Work out the finished part from the listing and answer in its coordinate system (mm). A direction names the side the tool comes from. Coordinates: 2 decimals unless noted, no trailing zeros. Order: outer loops, then holes, each group sorted by start corner. A loop starts at its lowest first (then second) coordinate and runs counter-clockwise, first axis right, second up. Notation, with made-up numbers: M -7.5,-28 L 40.5,-28 A16 ccw 40.5,-7 Z; hole C -30,-29 d7. An arc over 180 degrees is marked long. Answer in a Markdown table with one row per item. Add a question column.
Item 1: Flat-ended cylindrical pins translate along their axes: pin 1 Ø4 at (x, z) = (-9, 3.5) entering from -Y; pin 2 Ø4 at (x, y) = (13.5, -1.5) entering from +Z; pin 3 Ø3 at (x, y) = (17.145, 0) entering from -Z; pin 4 Ø2 at (y, z) = (0.5, 11.5) entering from +X (3 decimals). Find the tip coordinate at first contact, or state that the pin passes through.
Item 2: Which of the six approach directions +Z, -Z, +X, -X, +Y, -Y give full straight-line access (tool end or side, diameter ignored) to faces 1 (the face through (-5.3, -0.8, 7.3)), 2 (the face through (-12.657, -3.184, 3.393)), 3 (the face through (-4.191, 0, 10))?
Item 3: The part is cut by section A-A (z = 5.08). Write down the section's boundary in (x, y) (1 decimal), then the cut area to 3 significant figures.
Item 4: The part is cut by section B-B (y = 0.5). Write down the section's boundary in (x, z) (3 decimals).
Item 5: The part is cut by section C-C (x = -8.89). Write down the section's boundary in (y, z), then the cut area to 3 significant figures.
Item 6: The mould has two halves that part along X. Classify faces 4 (the face through (15, 0, 0)), 5 (the face through (-17.145, 0, 5)), 6 (the face through (-4.651, 0.053, 6.773)), 7 (the face through (20.954, -0.084, 5.009)): released by +X, released by -X, zero draft, split by the parting line, or undercut.
Item 7: Consider line 1 (Y direction, x = 17, z = 7.75); line 2 (X direction, y = 0.5, z = 11) (3 decimals); line 3 (Z direction, x = 8.5, y = 2.5). Determine where each line is inside the solid, lowest interval first. Write a range as from..to.
Item 8: The part is cut by section D-D (x = 11.5). Write down the section's boundary in (y, z).
from build123d import *

# Parameters (mm, degrees)
BOSS_EXTRUDE1_DEPTH   = 10.16
F_4_CLEARANCE_HOLE1_D = 3.4544
SKETCH4_R             = 1.905
CUT_EXTRUDE1_DEPTH    = 8.62
CUT_EXTRUDE1_TAPER    = -20
SKETCH5_R             = 4.1275
CUT_EXTRUDE2_DEPTH    = 1.27
SKETCH6_W             = 25.4
SKETCH6_H             = 2.54
BOSS_EXTRUDE2_DEPTH   = 7.62
CUT_EXTRUDE3_DEPTH    = 8.62


with BuildPart() as part:
    # Sketch1 → Boss-Extrude1 (new body)
    with BuildSketch(Plane.XY):
        with BuildLine():
            Line((-17.145, -3.81), (17.145, -3.81))
            ThreePointArc((17.145, -3.81), (20.955, 0), (17.145, 3.81))
            Line((17.145, 3.81), (-17.145, 3.81))
            Line((-17.145, 3.81), (-17.145, -3.81))
        make_face()
    extrude(amount=BOSS_EXTRUDE1_DEPTH)

    # #4 Clearance Hole1 (through all)
    with Locations(Plane.XY.offset(10.16)):
        with Locations((17.145, 0)):
            Hole(F_4_CLEARANCE_HOLE1_D / 2)

    # Sketch4 → Cut-Extrude1 (cut, through all)
    with BuildSketch(Plane(origin=(0, -3.81, 0), x_dir=(1, 0, 0), z_dir=(0, 1, 0))):
        with Locations((-8.89, -5.08)):
            Circle(SKETCH4_R)
    extrude(amount=CUT_EXTRUDE1_DEPTH, taper=CUT_EXTRUDE1_TAPER, mode=Mode.SUBTRACT)

    # Sketch5 → Cut-Extrude2 (cut)
    with BuildSketch(Plane.XZ.offset(3.81)):
        with Locations((-8.89, 5.08)):
            Circle(SKETCH5_R)
    extrude(amount=-CUT_EXTRUDE2_DEPTH, mode=Mode.SUBTRACT)

    # Sketch6 → Boss-Extrude2 (add, through all)
    with BuildSketch(Plane.XZ.offset(3.81)):
        with Locations((-4.445, 11.43)):
            Rectangle(SKETCH6_W, SKETCH6_H)
        with Locations((-4.445, -1.27)):
            Rectangle(SKETCH6_W, SKETCH6_H)
    extrude(amount=-BOSS_EXTRUDE2_DEPTH)

    # Sketch8 → Cut-Extrude3 (cut, through all)
    with BuildSketch(Plane(origin=(0, 3.81, 0), x_dir=(1, 0, 0), z_dir=(0, 1, 0))):
        Polygon((-3.429, -12.7), (-3.429, -7.38452905), (-8.71961162, -4.73922324), (-9.06038838, -5.42077676), (-4.191, -7.85547095), (-4.191, -12.7), align=None)
    extrude(amount=-CUT_EXTRUDE3_DEPTH, mode=Mode.SUBTRACT)


solid = part.part
Reply:
| question | item | result |
|---|---|---|
| 1 | pin 1 | stops at y = -2.54 |
| 1 | pin 2 | stops at z = 10.16 |
| 1 | pin 3 | passes through |
| 1 | pin 4 | stops at x = 8.255 |
| 2 | face 1 | +Y, -Y |
| 2 | face 2 | -Y |
| 2 | face 3 | +Z, +Y, -Y |
| 3 | outline | M -17.1,-3.8 L -13,-3.8 L -13,-2.5 L -11.3,-2.5 L -13.6,3.8 L -17.1,3.8 Z; M -6.5,-2.5 L -4.8,-2.5 L -4.8,-3.8 L 17.1,-3.8 A3.8 ccw 17.1,3.8 L -4.2,3.8 Z; hole C 17.1,0 d3.5 |
| 3 | area | 219 mm2 |
| 4 | outline | M -17.145,-2.54 L 8.255,-2.54 L 8.255,0 L 15.492,0 L 15.492,10.16 L 8.255,10.16 L 8.255,12.7 L -3.429,12.7 L -3.429,7.385 L -5.631,6.283 A3.474 cw long -5.972,6.965 L -4.191,7.855 L -4.191,12.7 L -17.145,12.7 Z; M 18.798,0 L 20.922,0 L 20.922,10.16 L 18.798,10.16 Z |
| 5 | outline | M -3.81,-2.54 L 3.81,-2.54 L 3.81,0.4 L -2.54,2.71 L -2.54,0.95 L -3.81,0.95 Z; M -3.81,9.21 L -2.54,9.21 L -2.54,7.45 L 3.81,9.76 L 3.81,12.7 L -3.81,12.7 Z |
| 5 | area | 60.9 mm2 |
| 6 | face 4 | zero draft |
| 6 | face 5 | released by -X |
| 6 | face 6 | undercut |
| 6 | face 7 | released by +X |
| 7 | line 1 | y = -3.81..-1.72, 1.72..3.81 |
| 7 | line 2 | x = -17.145..-4.191, -3.429..8.255 |
| 7 | line 3 | z = 0..10.16 |
| 8 | outline | M -3.81,0 L 3.81,0 L 3.81,10.16 L -3.81,10.16 Z |
